The model under review builds one solid part; all positions refer to its coordinate system, in mm. A direction names the side the tool comes from. Round coordinates to 2 decimals unless told otherwise and drop trailing zeros. Order: outer loops, then holes, each group sorted by start corner. A loop starts at its lowest first (then second) coordinate and runs counter-clockwise, first axis right, second up. Notation, with made-up numbers: M 17.5,16 L 44.5,16 A17 ccw 44.5,32 Z; hole C 85,25.5 d2. An arc over 180 degrees is marked long. Use a Markdown table: item, result. Add a question column.
1. Consider section C-C on z = 4. State the section outline as (x, y) points.
2. Consider section B-B on x = 25.4. State the section outline as (y, z) points, then the cut area to 3 significant figures.
3. Consider section A-A on y = -12.7. State the section outline as (x, z) points.
4. For faces 5 (the cylindrical face through (6.439, -12.894, 31.435)), 6 (the flat face through (34, -13, 12.7)), list the 3-axis set-ups (+Z, -Z, +X, -X, +Y, -Y) from which the entire face can be reached by the end or side of a thin tool; tool diameter is ignored.
5. Insertion check: P1, Ø12.5, axis at y = -11, z = 34, coming from the +X side; P2, Ø3, axis at y = -10, z = 5.5, coming from the +X side. Each pin has a flat end and moves straight along its axis. Give the tip position at first contact, or say it passes through.
6. To check wall thickness, follow probe 1 along Y at (x, z) = (44, 3); probe 2 along X at (y, z) = (-19.5, 25). State the ranges of each line that lie inside material, in increasing order.
7. Consider section D-D on z = 33.5. State the section outline as (x, y) points.
8. The part is to be moulded in two halves that separate along X. For faces 1 (the flat face through (0, -13, 17)), 2 (the cylindrical face through (50.316, -15.132, 6.439)), 3 (the cylindrical face through (20.36, -16.56, 6.44)), 4 (the cylindrical face through (6.439, -1.911, 42.754)), say which applies: +X half, -X half, draft (parallel to the pull), parting line (faces both ways), or undercut.
from build123d import *

# Parameters (mm, degrees)
F0_W      = 57.15
F0_H      = 44.45
F1_DEPTH  = 25.4
F2_W      = 44.45
F2_H      = 31.75
F3_DEPTH  = 25.4
F5_DEPTH  = 25.4
F7_DEPTH  = 25.4
F9_DEPTH  = 25.4
F10_R     = 6.35
F11_DEPTH = 25.4
F13_DEPTH = 25.4


with BuildPart() as f1:
    # F0 (on Front) → F1 (new body)
    with BuildSketch(Plane.XZ):
        with Locations((28.575, 22.225)):
            Rectangle(F0_W, F0_H)
    extrude(amount=F1_DEPTH)

    # F2 (on face) → F3 (cut)
    with BuildSketch(Plane.XZ.offset(25.4)):
        with Locations((34.925, 28.575)):
            Rectangle(F2_W, F2_H)
    extrude(amount=-F3_DEPTH, mode=Mode.SUBTRACT)

    # F4 (on face) → F5 (cut)
    with BuildSketch(Plane.YZ.offset(12.7)):
        with BuildLine():
            ThreePointArc((-19.049607, 37.71184), (-12.735329, 44.132399), (-6.35, 37.782498))
            ThreePointArc((-6.35, 37.782498), (-6.350663, 37.690749), (-6.352651, 37.59902))
            Line((-6.352651, 37.59902), (-6.154615, 44.45))
            Line((-6.154615, 44.45), (-19.124588, 44.45))
            Line((-19.124588, 44.45), (-19.049607, 37.71184))
        make_face()
        with BuildLine():
            ThreePointArc((-6.352651, 37.59902), (-6.350663, 37.690749), (-6.35, 37.782498))
            ThreePointArc((-6.35, 37.782498), (-12.735329, 44.132399), (-19.049607, 37.71184))
            ThreePointArc((-19.049607, 37.71184), (-12.756422, 31.432748), (-6.352651, 37.59902))
        make_face()
    extrude(amount=-F5_DEPTH, mode=Mode.SUBTRACT)

    # F6 (on face) → F7 (cut)
    with BuildSketch(Plane.YZ.offset(12.7)):
        with BuildLine():
            ThreePointArc((-25.4, 38.466346), (-23.46005, 42.71433), (-19.124588, 44.45))
            Line((-19.124588, 44.45), (-25.4, 44.45))
            Line((-25.4, 44.45), (-25.4, 38.466346))
        make_face()
    extrude(amount=-F7_DEPTH, mode=Mode.SUBTRACT)

    # F8 (on face) → F9 (cut)
    with BuildSketch(Plane.YZ.offset(12.7)):
        with BuildLine():
            ThreePointArc((-6.154615, 44.45), (-1.862663, 42.707521), (0, 38.466346))
            Line((0, 38.466346), (0, 44.45))
            Line((0, 44.45), (-6.154615, 44.45))
        make_face()
    extrude(amount=-F9_DEPTH, mode=Mode.SUBTRACT)

    # F10 (on face) → F11 (cut)
    with BuildSketch(Plane.XY.offset(12.7)):
        with Locations((44.45, -12.7)):
            Circle(F10_R)
        with Locations((25.4, -12.7)):
            Circle(F10_R)
    extrude(amount=-F11_DEPTH, mode=Mode.SUBTRACT)

    # F12 (on face) → F13 (cut)
    with BuildSketch(Plane.XY.offset(12.7)):
        with BuildLine():
            ThreePointArc((49.920771, 0), (56.759721, -12.7), (49.920771, -25.4))
            Line((49.920771, -25.4), (57.15, -25.4))
            Line((57.15, -25.4), (57.15, 0))
            Line((57.15, 0), (49.920771, 0))
        make_face()
    extrude(amount=-F13_DEPTH, mode=Mode.SUBTRACT)


solid = f1.part
Answer block:
| question | item | result |
|---|---|---|
| 1 | outline | M 0,-25.4 L 49.92,-25.4 A15.21 ccw 49.92,0 L 0,0 Z; hole C 25.4,-12.7 d12.7; hole C 44.45,-12.7 d12.7 |
| 2 | outline | M -25.4,0 L -19.05,0 L -19.05,12.7 L -25.4,12.7 Z; M -6.35,0 L 0,0 L 0,12.7 L -6.35,12.7 Z |
| 2 | area | 161 mm^2 |
| 3 | outline | M 0,0 L 19.05,0 L 19.05,12.7 L 12.7,12.7 L 12.7,31.43 L 0,31.43 Z; M 31.75,0 L 38.1,0 L 38.1,12.7 L 31.75,12.7 Z; M 50.8,0 L 56.76,0 L 56.76,12.7 L 50.8,12.7 Z |
| 4 | face 5 | +Z, +X, -X |
| 4 | face 6 | +Z, +X, +Y, -Y |
| 5 | P1 | x = 12.7 |
| 5 | P2 | x = 56.71 |
| 6 | probe 1 | -25.4 to -19.03, -6.37 to 0 |
| 6 | probe 2 | 0 to 12.7 |
| 7 | outline | M 0,-25.4 L 12.7,-25.4 L 12.7,-17.39 L 0,-17.39 Z; M 0,-8.01 L 12.7,-8.01 L 12.7,0 L 0,0 Z |
| 8 | face 1 | -X half |
| 8 | face 2 | undercut |
| 8 | face 3 | undercut |
| 8 | face 4 | draft |
